Autodesk Inventor part; units mm, degrees
ref_plane "YZ Plane" through (0, 0, 0) normal (1, 0, 0) x (0, 1, 0)
ref_plane "XZ Plane" through (0, 0, 0) normal (0, 1, 0) x (-1, 0, 0)
ref_plane "XY Plane" through (0, 0, 0) normal (0, 0, 1) x (1, 0, 0)
sketch "Sketch1" plane through (0, 0, 0) normal (0, 0, 1) x (1, 0, 0)
  circle A0 centre (0, 0) radius 31.75
  dimension "d0" = 63.5
extrude "Extrusion1" add sketch "Sketch1" along normal blind 286.0294
sketch "Sketch2" plane through (0, 0, 286.0294) normal (0, 0, 1) x (1, 0, 0)
  circle A0 centre (0, 0) radius 31.75
  circle A1 centre (0, 0) radius 14.5034
  dimension "d3" = 29.0068
extrude "Extrusion2" add sketch "Sketch2" along normal blind 8.3566 contours A1
sketch "Sketch3" plane through (0, 0, 0) normal (0, 0, -1) x (-1, 0, 0)
  circle A0 centre (0, 0) radius 31.75
  circle A1 centre (0, 0) radius 14.5034
  dimension "d6" = 29.0068
extrude "Extrusion3" add sketch "Sketch3" along normal blind 8.3566 contours A1
fillet "Fillet1" radius 12.7 2 edges at (-31.75, 0, 0) (-31.75, 0, 286.0294)
shell "Shell1" thickness 6.35 removed faces 2 at (0.6824, -3.9787, -8.3566) at (-0.6824, -3.9787, 294.386)
properties part number "Pneuare Tank" material "Polypropylene"
Source: CAD feature listing. Evaluate the final solid. Frame: model axes, mm. A direction names the side the tool comes from. Coordinates: 2 decimals unless noted, no trailing zeros. Write each loop counter-clockwise with the first axis right and the second up, starting at its lowest first coordinate (ties: lowest second). Pieces come first, ordered by that corner, then holes. Notation, with made-up numbers: M -36.75,45.5 L -4.75,45.5 A26 ccw -4.75,76.5 Z; hole C -39.5,-18 d11. An arc over 180 degrees is marked long. Answer as a JSON object with one key per item and string values.
1. Contact query for flat-ended pins moving along their axis: P1, Ø8, axis at x = 0, z = 205, coming from the +Y side; P2, Ø8, axis at x = -16.5, y = 13, coming from the -Z side; P3, Ø1.5, axis at x = -16.5, y = -17.5, coming from the -Z side. Output: stop coordinate, or through.
Evaluation:
{"P1": "y = 31.75", "P2": "z = 0", "P3": "z = 0.73"}
2. Draft query along Y for faces 4 (the flat face through (-4.32, -14.02, 286.029)), 5 (the cylindrical face through (-5.506, 24.796, 141.19)), 6 (the cylindrical face through (1.061, -8.084, -0.9)), 7 (the cylindrical face through (13.834, -4.356, 290.149)). Return one class per face: released by +Y, released by -Y, zero draft, split by the parting line, or undercut.
Evaluation:
{"face 4": "zero draft", "face 5": "undercut", "face 6": "undercut", "face 7": "split by the parting line"}
3. Ray query, L1, parallel to Y at x = 0, z = 132; L2, parallel to X at y = -1.5, z = 150; L3, parallel to Z at x = 3.5, y = -8.5. Return the intervals inside material, ascending.
Evaluation:
{"L1": "-31.75 to -25.4, 25.4 to 31.75", "L2": "-31.71 to -25.36, 25.36 to 31.71", "L3": "-8.36 to 6.35, 279.68 to 294.39"}
4. Cut plane C-C on z = 48. Output: boundary loops of the cut face in (x, y), plus the area to 3 significant figures.
Evaluation:
{"outline": "C 0,0 d63.5; hole C 0,0 d50.8", "area": "1,140 mm^2"}
5. Access query for faces 1 (the flat face through (8, -4, 279.679)), 2 (the cylindrical face through (-1.061, -8.084, 286.93)), 3 (the cylindrical face through (-13.834, -4.356, -4.12)). Directions: +Z, -Z, +X, -X, +Y, -Y. A direction counts if a zero-diameter tool reaches every point of the face in a straight line with its end or side. Return the directions, or none.
Evaluation:
{"face 1": "none", "face 2": "+Z, -Z", "face 3": "-Z"}
